Can you work these out from the drawing? Everything is in mm from the part's minimum corner. Give positions to 0.01 mm unless a question says otherwise; leave off trailing zeros. Write each loop counter-clockwise with the first axis right and the second up, starting at its lowest first coordinate (ties: lowest second). Pieces come first, ordered by that corner, then holes. Notation, with made-up numbers: (77.5, 40) -> (100.5, 40) arc R37 ccw to (100.5, 79) -> close; hole circle Ø11 at (65.5, 55.25). An arc over 180 degrees is marked (long way). Return JSON: item names as keys, results as strings.
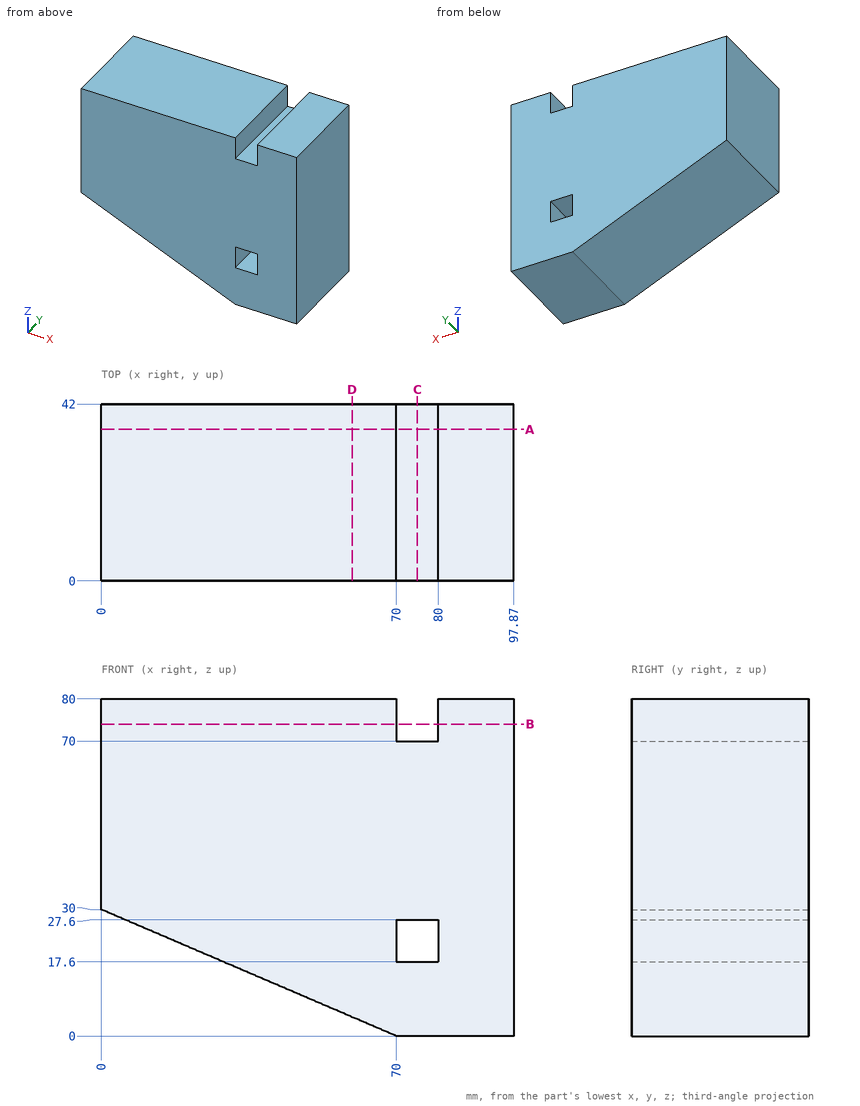
1. Suppose I cut it at B-B, the plane z = 74. List the corners of the cut face in (x, y) for me.
Taken from the geometry:
{"outline": "(0, 0) -> (70, 0) -> (70, 42) -> (0, 42) -> close; (80, 0) -> (97.87, 0) -> (97.87, 42) -> (80, 42) -> close"}
2. For pin 1 Ø2 at (y, z) = (19, 12) entering from -X; pin 2 Ø3 at (y, z) = (15, 23.5) entering from -X; pin 3 Ø3 at (x, y) = (75, 27) entering from +Z, each with a flat end and sliding along its axis, tell me the tip position at first contact or that it passes through.
Taken from the geometry:
{"pin 1": "stops at x = 39.67", "pin 2": "stops at x = 11.67", "pin 3": "stops at z = 70"}
3. Suppose I cut it at C-C, the plane x = 75. List the corners of the cut face in (y, z) for me.
Taken from the geometry:
{"outline": "(0, 0) -> (42, 0) -> (42, 17.6) -> (0, 17.6) -> close; (0, 27.6) -> (42, 27.6) -> (42, 70) -> (0, 70) -> close"}
4. If I drill on line 1 (X direction, y = 9, z = 22.5); line 2 (X direction, y = 2, z = 72); line 3 (Z direction, x = 68, y = 6), over which ranges is the centre line in solid material (lowest first)? Write a range as [from, to].
Taken from the geometry:
{"line 1": "x = [17.5, 70], [80, 97.87]", "line 2": "x = [0, 70], [80, 97.87]", "line 3": "z = [0.86, 80]"}
5. Suppose I cut it at D-D, the plane x = 59.5. List the corners of the cut face in (y, z) for me.
Taken from the geometry:
{"outline": "(0, 4.5) -> (42, 4.5) -> (42, 80) -> (0, 80) -> close"}
6. Suppose I cut it at A-A, the plane y = 36. List the corners of the cut face in (x, z) for me.
Taken from the geometry:
{"outline": "(0, 30) -> (70, 0) -> (97.87, 0) -> (97.87, 80) -> (80, 80) -> (80, 70) -> (70, 70) -> (70, 80) -> (0, 80) -> close; hole (70, 17.6) -> (80, 17.6) -> (80, 27.6) -> (70, 27.6) -> close"}
